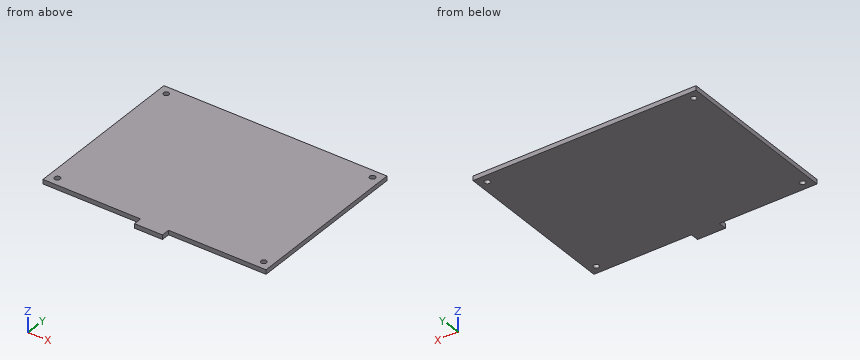
```python
from build123d import *

# Parameters (mm, degrees)
SKETCH_1_W      = 80
SKETCH_1_H      = 60
SKETCH_1_R      = 1
SKETCH_1_W_2    = 10
SKETCH_1_H_2    = 3
EXTRUDE_1_DEPTH = 1.6


with BuildPart() as part:
    # 草图1 → 凸台-拉伸1 (new body)
    # profile 1 of 2: a face of its own
    with BuildSketch(Plane.XY):
        Rectangle(SKETCH_1_W, SKETCH_1_H)
        with Locations((-37, 27)):
            Circle(SKETCH_1_R, mode=Mode.SUBTRACT)
        with Locations((37, 27)):
            Circle(SKETCH_1_R, mode=Mode.SUBTRACT)
        with Locations((37, -27)):
            Circle(SKETCH_1_R, mode=Mode.SUBTRACT)
        with Locations((-37, -27)):
            Circle(SKETCH_1_R, mode=Mode.SUBTRACT)
    # profile 2 of 2: a face of its own
    with BuildSketch(Plane.XY):
        with Locations((0, -31.5)):
            Rectangle(SKETCH_1_W_2, SKETCH_1_H_2)
    extrude(amount=EXTRUDE_1_DEPTH)


solid = part.part
```
Check sheet for the modelled part. Datum: model origin and axes. Units: mm. Give positions to 0.01 mm unless a question says otherwise; leave off trailing zeros. Order: outer loops, then holes, each group sorted by start corner. A loop starts at its lowest first (then second) coordinate and runs counter-clockwise, first axis right, second up. Notation, with made-up numbers: M 59,10.5 L 95,10.5 A20 cw 95,16.5 Z; hole C 11.25,14 d8. An arc over 180 degrees is marked long. Answer in a Markdown table with one row per item. Add a question column.
Q1. Sectioned sample at A-A, the plane z = 0.65. Record the boundary of the cut face in (x, y).
Q2. Sectioned sample at B-B, the plane y = 27. Record the boundary of the cut face in (x, z).
Q3. Thickness scan on L1, parallel to Y at x = -37, z = 0.6; L2, parallel to X at y = 27.5, z = 1.05; L3, parallel to Y at x = 10.5, z = 0.4. Record the ranges inside material, lowest first.
Q4. Sectioned sample at C-C, the plane x = -8.5. Record the boundary of the cut face in (y, z).
Q5. Gauge pin test, flat ends, axial feed: pin 1 Ø1.8 at (x, y) = (37, -27) entering from +Z; pin 2 Ø0.5 at (x, z) = (-24.5, 0.5) entering from -Y; pin 3 Ø0.5 at (y, z) = (-31, 1) entering from -X. Record the tip position at first contact, or that the pin passes through.
Verdict:
| question | item | result |
|---|---|---|
| 1 | outline | M -40,-30 L -5,-30 L -5,-33 L 5,-33 L 5,-30 L 40,-30 L 40,30 L -40,30 Z; hole C -37,-27 d2; hole C -37,27 d2; hole C 37,-27 d2; hole C 37,27 d2 |
| 2 | outline | M -40,0 L -38,0 L -38,1.6 L -40,1.6 Z; M -36,0 L 36,0 L 36,1.6 L -36,1.6 Z; M 38,0 L 40,0 L 40,1.6 L 38,1.6 Z |
| 3 | L1 | -30 to -28, -26 to 26, 28 to 30 |
| 3 | L2 | -40 to -37.87, -36.13 to 36.13, 37.87 to 40 |
| 3 | L3 | -30 to 30 |
| 4 | outline | M -30,0 L 30,0 L 30,1.6 L -30,1.6 Z |
| 5 | pin 1 | through |
| 5 | pin 2 | y = -30 |
| 5 | pin 3 | x = -5 |
